Geometry: final body of the model. Coordinates: model frame, mm. Face numbers are marked on the shaded views. A direction names the side the tool comes from. Give positions to 0.01 mm unless a question says otherwise; leave off trailing zeros. Loops run counter-clockwise (first coordinate to the right, second up) from the corner with the lowest first, then second, coordinate; pieces in that order, holes last.
1. Section B-B, the plane y = 10. Output: boundary loops of the cut face in (x, z), then the cut area to 3 significant figures.
2. Material intervals for line 1 along Y through (x, z) = (6.25, 8); line 2 along Y through (x, z) = (9.5, 2.5); line 3 along Z through (x, y) = (-0.5, 2.75), sorted ascending.
3. Draft query along X for the marked faces 1, 2 and 3. Return one class per face: +X half, -X half, draft (parallel to the pull), parting line (faces both ways), or undercut.
4. Section A-A, the plane x = 0. Output: boundary loops of the cut face in (y, z), then the cut area to 3 significant figures.
5. First-contact query: P1, Ø7, axis at x = 1.5, y = -3, coming from the -Z side; P2, Ø8, axis at x = 7.5, z = 27, coming from the -Y side; P3, Ø1.5, axis at x = -8, z = 9.5, coming from the +Y side. Flat tips, straight axial feed; report the tip coordinate or a pass-through.
6. Section C-C, the plane z = 29. Output: boundary loops of the cut face in (x, y), then the cut area to 3 significant figures.
7. Access query for the marked faces 4, 5 and 6. Directions: +Z, -Z, +X, -X, +Y, -Y. A direction counts if a zero-diameter tool reaches every point of the face in a straight line with its end or side. Return the directions, or none.
from build123d import *

# Parameters (mm, degrees)
SKETCH_1_R               = 13
EXTRUDE_1_DEPTH          = 10
CUT_EXTRUDE_START        = -10
CUT_EXTRUDE_1_DEPTH      = 10
PATTERN_CIRCULAR_3_COUNT = 11
SKETCH_3_R               = 7.5
CUT_EXTRUDE_2_DEPTH      = 4
CUT_EXTRUDE_2_DRAFT      = -6
SKETCH_4_R               = 7.5
CUT_EXTRUDE_3_DEPTH      = 4
CUT_EXTRUDE_3_DRAFT      = -6
SKETCH_5_R               = 4
EXTRUDE_2_DEPTH          = 30
CHAMFER_1_SIZE           = 1


with BuildPart() as part:
    # Эскиз1 → Бобышка-Вытянуть1 (new body)
    with BuildSketch(Plane.XY):
        Circle(SKETCH_1_R)
    extrude(amount=EXTRUDE_1_DEPTH)

    # Эскиз2 → Вырез-Вытянуть1 (cut)
    with BuildSketch(Plane.XY.offset(10).offset(CUT_EXTRUDE_START)):
        with BuildLine():
            ThreePointArc((1.252557909, 8.912412619), (0, 9), (-1.252557909, 8.912412619))
            ThreePointArc((-1.252557909, 8.912412619), (-1.684886314, 10.969320472), (-2.924363706, 12.666810842))
            ThreePointArc((-2.924363706, 12.666810842), (0, 13), (2.924363706, 12.666810842))
            ThreePointArc((2.924363706, 12.666810842), (1.684886314, 10.969320472), (1.252557909, 8.912412619))
        make_face()
    cut_extrude_1 = extrude(amount=CUT_EXTRUDE_1_DEPTH, mode=Mode.SUBTRACT)

    # Круговой массив3: Вырез-Вытянуть1 ×11 about axis
    pattern_circular_3_axis = Axis((0, 0, 0), (0, 0, 1))
    for i in range(1, PATTERN_CIRCULAR_3_COUNT):
        add(cut_extrude_1.rotate(pattern_circular_3_axis, i * 360 / PATTERN_CIRCULAR_3_COUNT), mode=Mode.SUBTRACT)


with BuildPart() as cut_extrude_2_tool:
    # Эскиз3 → Вырез-Вытянуть2 (with draft: the straight prism first)
    with BuildSketch(Plane.XY.offset(10)):
        Circle(SKETCH_3_R)
    extrude(amount=-CUT_EXTRUDE_2_DEPTH)
    # Вырез-Вытянуть2: the draft: its side faces are tilted about the plane it starts from
    cut_extrude_2_sides = [cut_extrude_2_tool.faces().sort_by_distance(p)[0] for p in [
        (-7.5, 0, 8),
    ]]
    draft(cut_extrude_2_sides, Plane.XY.offset(10), CUT_EXTRUDE_2_DRAFT)


with BuildPart() as part_1:
    add(part.part)

    # Вырез-Вытянуть2: cut by cut_extrude_2_tool
    add(cut_extrude_2_tool.part, mode=Mode.SUBTRACT)


with BuildPart() as cut_extrude_3_tool:
    # Эскиз4 → Вырез-Вытянуть3 (with draft: the straight prism first)
    with BuildSketch(Plane(origin=(0, 0, 0), x_dir=(-1, 0, 0), z_dir=(0, 0, -1))):
        Circle(SKETCH_4_R)
    extrude(amount=-CUT_EXTRUDE_3_DEPTH)
    # Вырез-Вытянуть3: the draft: its side faces are tilted about the plane it starts from
    cut_extrude_3_sides = [cut_extrude_3_tool.faces().sort_by_distance(p)[0] for p in [
        (7.5, 0, 2),
    ]]
    draft(cut_extrude_3_sides, Plane(origin=(0, 0, 0), x_dir=(-1, 0, 0), z_dir=(0, 0, -1)), CUT_EXTRUDE_3_DRAFT)


with BuildPart() as part_2:
    add(part_1.part)

    # Вырез-Вытянуть3: cut by cut_extrude_3_tool
    add(cut_extrude_3_tool.part, mode=Mode.SUBTRACT)

    # Эскиз5 → Бобышка-Вытянуть2 (add)
    with BuildSketch(Plane.XY.offset(6)):
        Circle(SKETCH_5_R)
    extrude(amount=EXTRUDE_2_DEPTH)

    # Фаска1
    chamfer_1_edges = [part_2.edges().sort_by_distance(p)[0] for p in [
        (-4, 0, 36),
    ]]
    chamfer(chamfer_1_edges, length=CHAMFER_1_SIZE)


solid = part_2.part
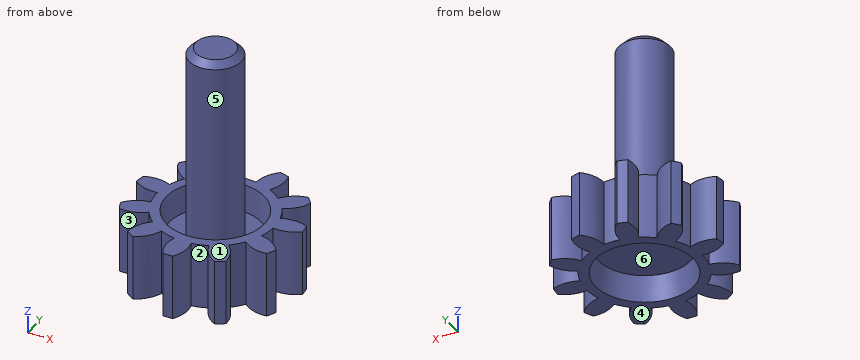
Answers below:
1. outline: (-4.49, 0) - (-1.37, 0) - (-1.37, 10) - (-4.49, 10) - close; (1.37, 0) - (4.49, 0) - (4.49, 10) - (1.37, 10) - close
1. area: 62.5 mm2
2. line 1: y = -11.27 to -7.1, -6.48 to -3.75, 3.75 to 7.34
2. line 2: y = -5.94 to -2.71, -0.08 to 2.87, 6.36 to 8.87
2. line 3: z = 4 to 36
3. face 1: draft
3. face 2: undercut
3. face 3: undercut
4. outline: (-13, 0) - (-7.5, 0) - (-7.08, 4) - (7.08, 4) - (7.5, 0) - (9, 0) - (9, 10) - (7.5, 10) - (7.08, 6) - (4, 6) - (4, 35) - (3, 36) - (-3, 36) - (-4, 35) - (-4, 6) - (-7.08, 6) - (-7.5, 10) - (-13, 10) - close
4. area: 342 mm2
5. P1: stops at z = 4
5. P2: stops at y = -1.94
5. P3: stops at y = 8.95
6. outline: circle Ø8 at (0, 0)
6. area: 50.3 mm2
7. face 4: -Z, +X, -X, +Y, -Y
7. face 5: +Z
7. face 6: -Z
